For this review, take the finished solid that the model builds, in its own axes (mm). A direction names the side the tool comes from. Give positions to 0.01 mm unless a question says otherwise; leave off trailing zeros. Order: outer loops, then holes, each group sorted by start corner. A loop starts at its lowest first (then second) coordinate and runs counter-clockwise, first axis right, second up. Notation, with made-up numbers: (-19, -12.5) -> (32, -12.5) arc R17 cw to (32, -7.5) -> close; hole circle Ø11 at (49, -12). An arc over 180 degrees is marked (long way). One line per item, written item: value. Start each with the question number.
from build123d import *

# Parameters (mm, degrees)
SKETCH1_W                                            = 38.1
SKETCH1_H                                            = 34.925
BOSS_EXTRUDE1_DEPTH                                  = 19.05
SKETCH3_W                                            = 38.1
SKETCH3_H                                            = 28.575
CUT_EXTRUDE1_DEPTH                                   = 28.575
CSK_FOR_M6_HEX_SOCKET_COUNTERSUNK_HEAD_S_D           = 6.4
CSK_FOR_M6_HEX_SOCKET_COUNTERSUNK_HEAD_S_CSINK_D     = 13.5
CSK_FOR_M6_HEX_SOCKET_COUNTERSUNK_HEAD_S_CSINK_ANGLE = 90


with BuildPart() as part:
    # Sketch1 → Boss-Extrude1 (new body, symmetric)
    with BuildSketch(Plane.XY):
        Rectangle(SKETCH1_W, SKETCH1_H)
    extrude(amount=BOSS_EXTRUDE1_DEPTH, both=True)

    # Sketch3 → Cut-Extrude1 (cut)
    with BuildSketch(Plane.XY.offset(19.05)):
        Rectangle(SKETCH3_W, SKETCH3_H)
    extrude(amount=-CUT_EXTRUDE1_DEPTH, mode=Mode.SUBTRACT)

    # CSK for M6 Hex Socket Countersunk Head Screw1 (through all)
    with Locations(Plane.XY.offset(-9.525)):
        with Locations((-11.43, 0), (11.43, 0)):
            CounterSinkHole(CSK_FOR_M6_HEX_SOCKET_COUNTERSUNK_HEAD_S_D / 2, CSK_FOR_M6_HEX_SOCKET_COUNTERSUNK_HEAD_S_CSINK_D / 2, counter_sink_angle=CSK_FOR_M6_HEX_SOCKET_COUNTERSUNK_HEAD_S_CSINK_ANGLE)


solid = part.part
Q1. Take a section at A-A (y = 0). State the section outline as (x, z) points (3 decimals), and give its area (3 significant figures).
Q2. Take a section at B-B (z = -4.5). State the section outline as (x, y) points.
Q3. For pin 1 Ø10 at (x, y) = (-11.43, 0) entering from +Z (3 decimals); pin 2 Ø3 at (x, y) = (3, 3.5) entering from +Z (3 decimals), all flat-tipped, find the tip position at first contact; note any pin that passes through.
Q4. Mouldability with a two-part tool opening along Y and no side actions: class faces 1 (the conical face through (-8.06, 0.15, -12.9)), 2 (the flat face through (0, -14.288, 5)), 3 (the flat face through (0, 17.462, 0)), 4 (the flat face through (0, 0, -19.05)) as pulls with the +Y half, pulls with the -Y half, needs draft (parallel to the pull), parting line crosses it, or undercut.
Q5. For line 1 along X through (y, z) = (0, -16.55); line 2 along Y through (x, z) = (9, -11); line 3 along Y through (x, z) = (7, -7), list the stretches that pass through material, from the lowest coordinate up.
Q6. For faces 5 (the flat face through (19.05, 0, -12)), 6 (the flat face through (0, 0, -9.525)), list the 3-axis set-ups (+Z, -Z, +X, -X, +Y, -Y) from which the entire face can be reached by the end or side of a thin tool; tool diameter is ignored.
Q7. Take a section at D-D (z = -15.5). State the section outline as (x, y) points, and give its area (3 significant figures).
Answers below:
1. outline: (-19.05, -19.05) -> (-14.63, -19.05) -> (-14.63, -13.075) -> (-18.18, -9.525) -> (-19.05, -9.525) -> close; (-8.23, -19.05) -> (8.23, -19.05) -> (8.23, -13.075) -> (4.68, -9.525) -> (-4.68, -9.525) -> (-8.23, -13.075) -> close; (14.63, -19.05) -> (19.05, -19.05) -> (19.05, -9.525) -> (18.18, -9.525) -> (14.63, -13.075) -> close
1. area: 216 mm²
2. outline: (-19.05, -17.46) -> (19.05, -17.46) -> (19.05, -14.29) -> (-19.05, -14.29) -> close; (-19.05, 14.29) -> (19.05, 14.29) -> (19.05, 17.46) -> (-19.05, 17.46) -> close
3. pin 1: stops at z = -11.275
3. pin 2: stops at z = -9.525
4. face 1: undercut
4. face 2: undercut
4. face 3: pulls with the +Y half
4. face 4: needs draft
5. line 1: x = -19.05 to -14.63, -8.23 to 8.23, 14.63 to 19.05
5. line 2: y = -17.46 to -4.68, 4.68 to 17.46
5. line 3: y = -17.46 to -14.29, 14.29 to 17.46
6. face 5: +Z, -Z, +X, +Y, -Y
6. face 6: +Z, +X, -X
7. outline: (-19.05, -17.46) -> (19.05, -17.46) -> (19.05, 17.46) -> (-19.05, 17.46) -> close; hole circle Ø6.4 at (-11.43, 0); hole circle Ø6.4 at (11.43, 0)
7. area: 1,270 mm²
